Could you check a few things on this model? Use its own coordinates, in mm. Face numbers are marked on the shaded views. Round coordinates to 2 decimals unless told otherwise and drop trailing zeros. Loops run counter-clockwise (first coordinate to the right, second up) from the corner with the lowest first, then second, coordinate; pieces in that order, holes last. Notation, with made-up numbers: (36, 1.25) - (46, 1.25) arc R11 ccw to (46, 14.25) - close; hole circle Ø5 at (35.5, 36). An arc over 180 degrees is marked (long way). Answer as CSV lines item,"result". Start each with the question number.
1) Suppose I cut it at B-B, the plane y = 27.5. Write out the boundary of the cut face in (x, z), then the cut area to 3 significant figures.
2) Please list where these lines run through material, in increasing order: line 1 along X through (y, z) = (0.75, -127); line 2 along Z through (x, y) = (863.6, 0.65); line 3 along Z through (x, y) = (-573, 39).
3) Suppose I cut it at C-C, the plane x = 477. Write out the boundary of the cut face in (y, z).
4) We'd pull the mould along Z, two halves only. Please class the marked faces 1 and 2: pulls with the +Z half, pulls with the -Z half, needs draft (parallel to the pull), parting line crosses it, or undercut.
5) Suppose I cut it at A-A, the plane z = 86. Write out the boundary of the cut face in (x, y) (3 decimals).
6) I'm going to push flat-ended pins straight in: pin 1 Ø8 at (x, z) = (901.7, -38.1) entering from +Y; pin 2 Ø3 at (x, z) = (733.5, -157) entering from -Y; pin 3 Ø1.3 at (x, y) = (78, 1) entering from -Z. Where does each tip first touch, or does it pass through?
```python
from build123d import *

# Parameters (mm, degrees)
SKETCH1_W                        = 1828.8
SKETCH1_H                        = 317.5
BOSS_EXTRUDE1_DEPTH              = 2.65684
CUT_EXTRUDE1_DEPTH               = 929.081882863
SKETCH3_R                        = 2.3876
CUT_EXTRUDE2_DEPTH               = 929.081882863
LPATTERN1_COUNT                  = 2
LPATTERN1_PITCH                  = 203.2
F_10_0_1935_DIAMETER_HOLE1_D     = 4.9149
F_10_0_1935_DIAMETER_HOLE1_DEPTH = 2.65684
F_10_0_1935_DIAMETER_HOLE2_D     = 4.9149
EDGE_FLANGE1_STRIP_W             = 15.94104
EDGE_FLANGE1_STRIP_H             = 2.65684
EDGE_FLANGE1_STRIP_CUT_DEPTH     = 1828.8
EDGE_FLANGE1_DEPTH               = 1828.8
EDGE_FLANGE2_STRIP_W             = 15.94104
EDGE_FLANGE2_STRIP_H             = 2.65684
EDGE_FLANGE2_STRIP_CUT_DEPTH     = 1828.8
EDGE_FLANGE2_DEPTH               = 1828.8
FILLET1_R                        = 12.7
CUT_EXTRUDE3_DEPTH               = 971.03394786
F_1_4_CLEARANCE_HOLE1_D          = 6.7564


# Sheet-metal steps are written as plain solids
with BuildPart() as part:
    # Sketch1 → Boss-Extrude1 (new body)
    with BuildSketch(Plane(origin=(0, 0, 0), x_dir=(1, 0, 0), z_dir=(0, 1, 0))):
        Rectangle(SKETCH1_W, SKETCH1_H)
    extrude(amount=BOSS_EXTRUDE1_DEPTH)

    # Sketch2 → Cut-Extrude1 (cut, through all)
    with BuildSketch(Plane(origin=(0, 2.65684, 0), x_dir=(1, 0, 0), z_dir=(0, 1, 0))):
        with BuildLine():
            Line((-104.775, 123.825), (-66.675, 123.825))
            ThreePointArc((-66.675, 123.825), (-62.184871939, 121.965128061), (-60.325, 117.475))
            Line((-60.325, 117.475), (-60.325, 53.975))
            ThreePointArc((-60.325, 53.975), (-62.184871939, 49.484871939), (-66.675, 47.625))
            Line((-66.675, 47.625), (-104.775, 47.625))
            ThreePointArc((-104.775, 47.625), (-109.265128061, 49.484871939), (-111.125, 53.975))
            Line((-111.125, 53.975), (-111.125, 117.475))
            ThreePointArc((-111.125, 117.475), (-109.265128061, 121.965128061), (-104.775, 123.825))
        make_face()
        with BuildLine():
            Line((-104.775, -47.625), (-66.675, -47.625))
            ThreePointArc((-66.675, -47.625), (-62.184871939, -49.484871939), (-60.325, -53.975))
            Line((-60.325, -53.975), (-60.325, -117.475))
            ThreePointArc((-60.325, -117.475), (-62.184871939, -121.965128061), (-66.675, -123.825))
            Line((-66.675, -123.825), (-104.775, -123.825))
            ThreePointArc((-104.775, -123.825), (-109.265128061, -121.965128061), (-111.125, -117.475))
            Line((-111.125, -117.475), (-111.125, -53.975))
            ThreePointArc((-111.125, -53.975), (-109.265128061, -49.484871939), (-104.775, -47.625))
        make_face()
        with BuildLine():
            Line((66.675, -47.625), (104.775, -47.625))
            ThreePointArc((104.775, -47.625), (109.265128061, -49.484871939), (111.125, -53.975))
            Line((111.125, -53.975), (111.125, -117.475))
            ThreePointArc((111.125, -117.475), (109.265128061, -121.965128061), (104.775, -123.825))
            Line((104.775, -123.825), (66.675, -123.825))
            ThreePointArc((66.675, -123.825), (62.184871939, -121.965128061), (60.325, -117.475))
            Line((60.325, -117.475), (60.325, -53.975))
            ThreePointArc((60.325, -53.975), (62.184871939, -49.484871939), (66.675, -47.625))
        make_face()
        with BuildLine():
            Line((104.775, 123.825), (66.675, 123.825))
            ThreePointArc((66.675, 123.825), (62.184871939, 121.965128061), (60.325, 117.475))
            Line((60.325, 117.475), (60.325, 53.975))
            ThreePointArc((60.325, 53.975), (62.184871939, 49.484871939), (66.675, 47.625))
            Line((66.675, 47.625), (104.775, 47.625))
            ThreePointArc((104.775, 47.625), (109.265128061, 49.484871939), (111.125, 53.975))
            Line((111.125, 53.975), (111.125, 117.475))
            ThreePointArc((111.125, 117.475), (109.265128061, 121.965128061), (104.775, 123.825))
        make_face()
    extrude(amount=-CUT_EXTRUDE1_DEPTH, mode=Mode.SUBTRACT)

    # Sketch3 → Cut-Extrude2 (cut, through all)
    with BuildSketch(Plane(origin=(0, 2.65684, 0), x_dir=(1, 0, 0), z_dir=(0, 1, 0))):
        with Locations(Location((-165.1, 127, 0), (0, 0, 270))):
            Circle(SKETCH3_R)
        with Locations(Location((-165.1, 0, 0), (0, 0, 270))):
            Circle(SKETCH3_R)
        with Locations(Location((-165.1, -127, 0), (0, 0, 270))):
            Circle(SKETCH3_R)
        with Locations(Location((-38.1, 127, 0), (0, 0, 270))):
            Circle(SKETCH3_R)
        with Locations(Location((-38.1, 0, 0), (0, 0, 270))):
            Circle(SKETCH3_R)
        with Locations(Location((-38.1, -127, 0), (0, 0, 270))):
            Circle(SKETCH3_R)
    cut_extrude2 = extrude(amount=-CUT_EXTRUDE2_DEPTH, mode=Mode.SUBTRACT)

    # LPattern1: Cut-Extrude2 ×2
    with Locations(*[(i * LPATTERN1_PITCH, 0, 0) for i in range(1, LPATTERN1_COUNT)]):
        add(cut_extrude2, mode=Mode.SUBTRACT)

    # #10 (0.1935) Diameter Hole1
    with Locations(Plane(origin=(0, 2.65684, 0), x_dir=(1, 0, 0), z_dir=(0, 1, 0))):
        with Locations((165.1, 127), (38.1, 127), (-38.1, 127), (165.1, 0), (165.1, -127), (-38.1, 0), (38.1, 0), (38.1, -127), (-38.1, -127), (-165.1, -127), (-165.1, 0), (-165.1, 127)):
            Hole(F_10_0_1935_DIAMETER_HOLE1_D / 2, depth=F_10_0_1935_DIAMETER_HOLE1_DEPTH)

    # #10 (0.1935) Diameter Hole2 (through all)
    with Locations(Plane(origin=(0, 2.65684, 0), x_dir=(1, 0, 0), z_dir=(0, 1, 0))):
        with Locations((901.7, 38.1), (863.6, 38.1), (825.5, 38.1), (825.5, -38.1), (863.6, -38.1), (901.7, -38.1)):
            f_10_0_1935_diameter_hole2 = Hole(F_10_0_1935_DIAMETER_HOLE2_D / 2)

    # Mirror1: #10 (0.1935) Diameter Hole2 across plane
    add(f_10_0_1935_diameter_hole2.mirror(Plane(origin=(0, 0, 0), x_dir=(0, 0, 1), z_dir=(1, 0, 0))), mode=Mode.SUBTRACT)

    # Edge-Flange1 strip (across the edge) → Edge-Flange1 strip cut (cut)
    with BuildSketch(Plane(origin=(914.4, 2.65684, -158.75), x_dir=(0, 0, 1), z_dir=(-1, 0, 0))):
        with Locations((-2.65684, -1.32842)):
            Rectangle(EDGE_FLANGE1_STRIP_W, EDGE_FLANGE1_STRIP_H)
    extrude(amount=EDGE_FLANGE1_STRIP_CUT_DEPTH, mode=Mode.SUBTRACT)

    # Edge-Flange1 section (across the edge) → Edge-Flange1 (add)
    with BuildSketch(Plane(origin=(914.4, 2.65684, -158.75), x_dir=(0, 0, 1), z_dir=(-1, 0, 0))):
        with BuildLine():
            Line((0, 2.65684), (0, 60.84316))
            Line((0, 60.84316), (2.65684, 60.84316))
            Line((2.65684, 60.84316), (2.65684, 2.65684))
            ThreePointArc((2.65684, 2.65684), (3.435010419, 0.778170419), (5.31368, 0))
            Line((5.31368, 0), (5.31368, -2.65684))
            ThreePointArc((5.31368, -2.65684), (1.556340839, -1.100499161), (0, 2.65684))
        make_face()
    extrude(amount=EDGE_FLANGE1_DEPTH)

    # Edge-Flange2 strip (across the edge) → Edge-Flange2 strip cut (cut)
    with BuildSketch(Plane(origin=(-914.4, 2.65684, 158.75), x_dir=(0, 0, -1), z_dir=(1, 0, 0))):
        with Locations((-2.65684, -1.32842)):
            Rectangle(EDGE_FLANGE2_STRIP_W, EDGE_FLANGE2_STRIP_H)
    extrude(amount=EDGE_FLANGE2_STRIP_CUT_DEPTH, mode=Mode.SUBTRACT)

    # Edge-Flange2 section (across the edge) → Edge-Flange2 (add)
    with BuildSketch(Plane(origin=(-914.4, 2.65684, 158.75), x_dir=(0, 0, -1), z_dir=(1, 0, 0))):
        with BuildLine():
            Line((0, 2.65684), (0, 60.84316))
            Line((0, 60.84316), (2.65684, 60.84316))
            Line((2.65684, 60.84316), (2.65684, 2.65684))
            ThreePointArc((2.65684, 2.65684), (3.435010419, 0.778170419), (5.31368, 0))
            Line((5.31368, 0), (5.31368, -2.65684))
            ThreePointArc((5.31368, -2.65684), (1.556340839, -1.100499161), (0, 2.65684))
        make_face()
    extrude(amount=EDGE_FLANGE2_DEPTH)

    # Fillet1
    fillet1_edges = [part.edges().sort_by_distance(p)[0] for p in [
        (914.4, 63.5, -157.42158),
        (-914.4, 63.5, -157.42158),
        (-914.4, 63.5, 157.42158),
        (914.4, 63.5, 157.42158),
    ]]
    fillet(fillet1_edges, radius=FILLET1_R)

    # Sketch21 → Cut-Extrude3 (cut, through all)
    with BuildSketch(Plane.XY.offset(158.75)):
        with BuildLine():
            Line((-819.15, 47.625), (-704.85, 47.625))
            ThreePointArc((-704.85, 47.625), (-688.975, 31.75), (-704.85, 15.875))
            Line((-704.85, 15.875), (-819.15, 15.875))
            ThreePointArc((-819.15, 15.875), (-835.025, 31.75), (-819.15, 47.625))
        make_face()
    cut_extrude3 = extrude(amount=-CUT_EXTRUDE3_DEPTH, mode=Mode.SUBTRACT)

    # 1/4 Clearance Hole1 (through all)
    with Locations(Plane(origin=(0, 0, -158.75), x_dir=(-1, 0, 0), z_dir=(0, 0, -1))):
        with Locations((904.875, 50.8), (904.875, 12.7)):
            f_1_4_clearance_hole1 = Hole(F_1_4_CLEARANCE_HOLE1_D / 2)

    # Mirror2: Cut-Extrude3, 1/4 Clearance Hole1 across plane
    add(cut_extrude3.mirror(Plane(origin=(0, 0, 0), x_dir=(0, 0, 1), z_dir=(1, 0, 0))), mode=Mode.SUBTRACT)
    add(f_1_4_clearance_hole1.mirror(Plane(origin=(0, 0, 0), x_dir=(0, 0, 1), z_dir=(1, 0, 0))), mode=Mode.SUBTRACT)


solid = part.part
```
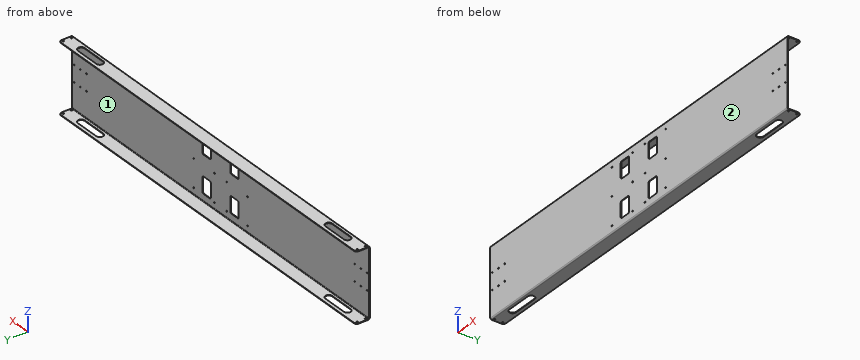
Filled sheet:
1,outline,"(-914.4, -158.75) - (-834.45, -158.75) - (-834.45, -156.09) - (-914.4, -156.09) - close; (-914.4, 156.09) - (-834.45, 156.09) - (-834.45, 158.75) - (-914.4, 158.75) - close; (-689.55, -158.75) - (689.55, -158.75) - (689.55, -156.09) - (-689.55, -156.09) - close; (-689.55, 156.09) - (689.55, 156.09) - (689.55, 158.75) - (-689.55, 158.75) - close; (834.45, -158.75) - (914.4, -158.75) - (914.4, -156.09) - (834.45, -156.09) - close; (834.45, 156.09) - (914.4, 156.09) - (914.4, 158.75) - (834.45, 158.75) - close"
1,area,"8,180 mm²"
2,line 1,"-914.4 to -167.56, -162.64 to -40.56, -35.64 to 35.64, 40.56 to 162.64, 167.56 to 914.4"
2,line 2,"-155.98 to -40.56, -35.64 to 35.64, 40.56 to 155.98"
2,line 3,"-158.75 to -156.09, 156.09 to 158.75"
3,outline,"(0, -153.44) arc R5.31 ccw to (5.31, -158.75) - (63.5, -158.75) - (63.5, -156.09) - (5.31, -156.09) arc R2.66 cw to (2.66, -153.44) - (2.66, 153.44) arc R2.66 cw to (5.31, 156.09) - (63.5, 156.09) - (63.5, 158.75) - (5.31, 158.75) arc R5.31 ccw to (0, 153.44) - close"
4,face 1,"undercut"
4,face 2,"needs draft"
5,outline,"(-914.4, 0) - (-111.125, 0) - (-111.125, 2.657) - (-914.4, 2.657) - close; (-60.325, 0) - (60.325, 0) - (60.325, 2.657) - (-60.325, 2.657) - close; (111.125, 0) - (914.4, 0) - (914.4, 2.657) - (111.125, 2.657) - close"
6,pin 1,"y = 2.66"
6,pin 2,"y = 0.42"
6,pin 3,"z = -157.29"
